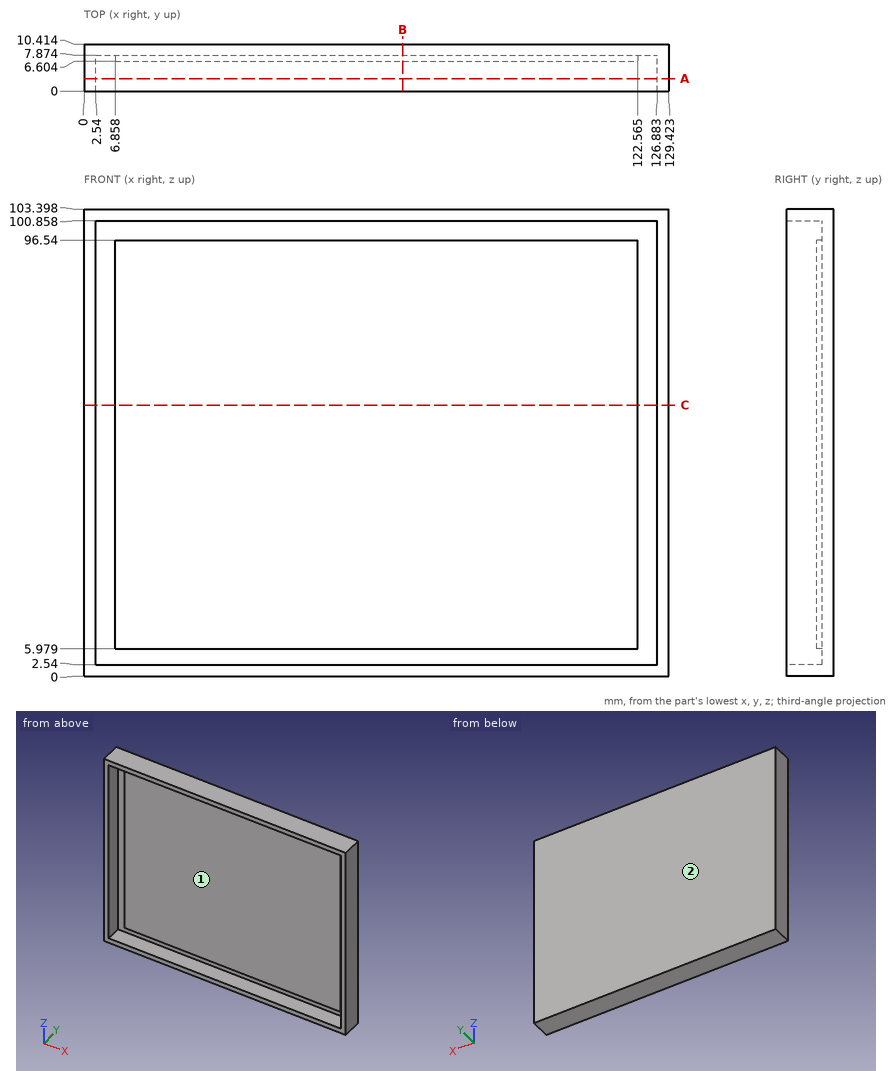
Drawing for the job (mm, zero at the part's lowest x, y, z). Give positions to 0.01 mm unless a question says otherwise; leave off trailing zeros. Loops run counter-clockwise (first coordinate to the right, second up) from the corner with the lowest first, then second, coordinate; pieces in that order, holes last.
1) Band-saw the part on C-C on z = 60. List the corners of the cut face in (x, y) (1 decimal).
Values follow:
outline: (0, 0) - (2.5, 0) - (2.5, 7.9) - (6.9, 7.9) - (6.9, 6.6) - (122.6, 6.6) - (122.6, 7.9) - (126.9, 7.9) - (126.9, 0) - (129.4, 0) - (129.4, 10.4) - (0, 10.4) - close
2) Probe line 1 along X through (y, z) = (2.75, 4); line 2 along Z through (x, y) = (76.5, 5.25); line 3 along Y through (x, z) = (11, 10). List the from-to ranges inside material, lowest first.
Values follow:
line 1: x = 0 to 2.54, 126.88 to 129.42
line 2: z = 0 to 2.54, 100.86 to 103.4
line 3: y = 6.6 to 10.41
3) Drop a flat-ended pin along its axis: P1, Ø1.5, axis at x = 21.5, z = 45.5, coming from the -Y side. Give the stop position or say it passes through.
Values follow:
P1: stops at y = 6.6
4) Band-saw the part on A-A on y = 2.75. List the corners of the cut face in (x, z), then the cut area to 3 significant figures.
Values follow:
outline: (0, 0) - (129.42, 0) - (129.42, 103.4) - (0, 103.4) - close; hole (2.54, 2.54) - (126.88, 2.54) - (126.88, 100.86) - (2.54, 100.86) - close
area: 1,160 mm2
5) Two-plate mould, pull along Z, no slides. Class the marked faces 1 and 2: released by +Z, released by -Z, zero draft, split by the parting line, or undercut.
Values follow:
face 1: undercut
face 2: zero draft
6) Band-saw the part on B-B on x = 70.5. List the corners of the cut face in (y, z).
Values follow:
outline: (0, 0) - (10.41, 0) - (10.41, 103.4) - (0, 103.4) - (0, 100.86) - (7.87, 100.86) - (7.87, 96.54) - (6.6, 96.54) - (6.6, 5.98) - (7.87, 5.98) - (7.87, 2.54) - (0, 2.54) - close
